from build123d import *

# Parameters (mm, degrees)
SKETCH_1_R      = 50
SKETCH_1_R_2    = 1.5
SKETCH_1_R_3    = 13.5
EXTRUDE_1_DEPTH = 3


with BuildPart() as part:
    # 草图1 → 凸台-拉伸1 (new body)
    with BuildSketch(Plane.XY):
        Circle(SKETCH_1_R)
        with Locations((0, 17)):
            Circle(SKETCH_1_R_2, mode=Mode.SUBTRACT)
        with Locations((17, 0)):
            Circle(SKETCH_1_R_2, mode=Mode.SUBTRACT)
        with Locations((0, -17)):
            Circle(SKETCH_1_R_2, mode=Mode.SUBTRACT)
        with Locations((-17, 0)):
            Circle(SKETCH_1_R_2, mode=Mode.SUBTRACT)
        with Locations((-23.461747754, 27.960622174)):
            Circle(SKETCH_1_R_2, mode=Mode.SUBTRACT)
        with Locations((0, 36.5)):
            Circle(SKETCH_1_R_2, mode=Mode.SUBTRACT)
        with Locations((23.461747754, 27.960622174)):
            Circle(SKETCH_1_R_2, mode=Mode.SUBTRACT)
        with Locations((35.945482985, 6.338158485)):
            Circle(SKETCH_1_R_2, mode=Mode.SUBTRACT)
        with Locations((31.609927238, -18.25)):
            Circle(SKETCH_1_R_2, mode=Mode.SUBTRACT)
        with Locations((12.483735231, -34.298780659)):
            Circle(SKETCH_1_R_2, mode=Mode.SUBTRACT)
        with Locations((-12.483735231, -34.298780659)):
            Circle(SKETCH_1_R_2, mode=Mode.SUBTRACT)
        with Locations((-31.609927238, -18.25)):
            Circle(SKETCH_1_R_2, mode=Mode.SUBTRACT)
        with Locations((-35.945482985, 6.338158485)):
            Circle(SKETCH_1_R_2, mode=Mode.SUBTRACT)
        Circle(SKETCH_1_R_3, mode=Mode.SUBTRACT)
    extrude(amount=EXTRUDE_1_DEPTH)


solid = part.part
CAD build for the part. Positions are in the model's coordinates, mm. Give positions to 0.01 mm unless a question says otherwise; leave off trailing zeros. Loops run counter-clockwise (first coordinate to the right, second up) from the corner with the lowest first, then second, coordinate; pieces in that order, holes last. Notation, with made-up numbers: M -18,-6 L 0,-6 A28 cw 0,33 Z; hole C 83,67 d7. An arc over 180 degrees is marked long. One line per question, with ' | ' between items. Start each with the question number.
1. Saw through at C-C on y = -10. Give the cut face in (x, z), plus the area to 3 significant figures.
2. Two-plate mould, pull along Y, no slides. Class faces 1 (the face through (10, -10, 3)), 2 (the face through (47.69, 15.02, 1.48)), 3 (the face through (-32.72, -17.24, 1.48)), 4 (the face through (-2.93, -13.18, 1.48)): pulls with the +Y half, pulls with the -Y half, needs draft (parallel to the pull), parting line crosses it, or undercut.
3. Probe L1, parallel to Y at x = 0, z = 2.25; L2, parallel to Y at x = -11.5, z = 0.95; L3, parallel to X at y = 7, z = 1.05. List the from-to ranges inside material, lowest first. Write a range as from..to.
4. Saw through at A-A on y = 0. Give the cut face in (x, z), plus the area to 3 significant figures.
5. Saw through at B-B on x = 0. Give the cut face in (y, z).
6. Flat gauge pins, fed straight in: pin 1 (2.5 mm diameter, centred on x = 35.95, y = 6.34, fed in from +Z); pin 2 (3.5 mm diameter, centred on x = -23.46, y = 27.96, fed in from +Z). Where does each tip first touch, or does it go through?
7. Saw through at D-D on z = 1.2. State how many separate pieces and enclosed holes the cut face has, plus the area to 3 significant figures.
Result sheet:
1) outline: M -48.99,0 L -9.07,0 L -9.07,3 L -48.99,3 Z; M 9.07,0 L 48.99,0 L 48.99,3 L 9.07,3 Z | area: 240 mm^2
2) face 1: needs draft | face 2: parting line crosses it | face 3: undercut | face 4: undercut
3) L1: y = -50..-18.5, -15.5..-13.5, 13.5..15.5, 18.5..35, 38..50 | L2: y = -48.66..-35.43, -33.17..-7.07, 7.07..48.66 | L3: x = -49.51..-37.29, -34.6..-11.54, 11.54..34.6, 37.29..49.51
4) outline: M -50,0 L -18.5,0 L -18.5,3 L -50,3 Z; M -15.5,0 L -13.5,0 L -13.5,3 L -15.5,3 Z; M 13.5,0 L 15.5,0 L 15.5,3 L 13.5,3 Z; M 18.5,0 L 50,0 L 50,3 L 18.5,3 Z | area: 201 mm^2
5) outline: M -50,0 L -18.5,0 L -18.5,3 L -50,3 Z; M -15.5,0 L -13.5,0 L -13.5,3 L -15.5,3 Z; M 13.5,0 L 15.5,0 L 15.5,3 L 13.5,3 Z; M 18.5,0 L 35,0 L 35,3 L 18.5,3 Z; M 38,0 L 50,0 L 50,3 L 38,3 Z
6) pin 1: passes through | pin 2: stops at z = 3
7) separate pieces: 1 | enclosed holes: 14 | area: 7,190 mm^2
